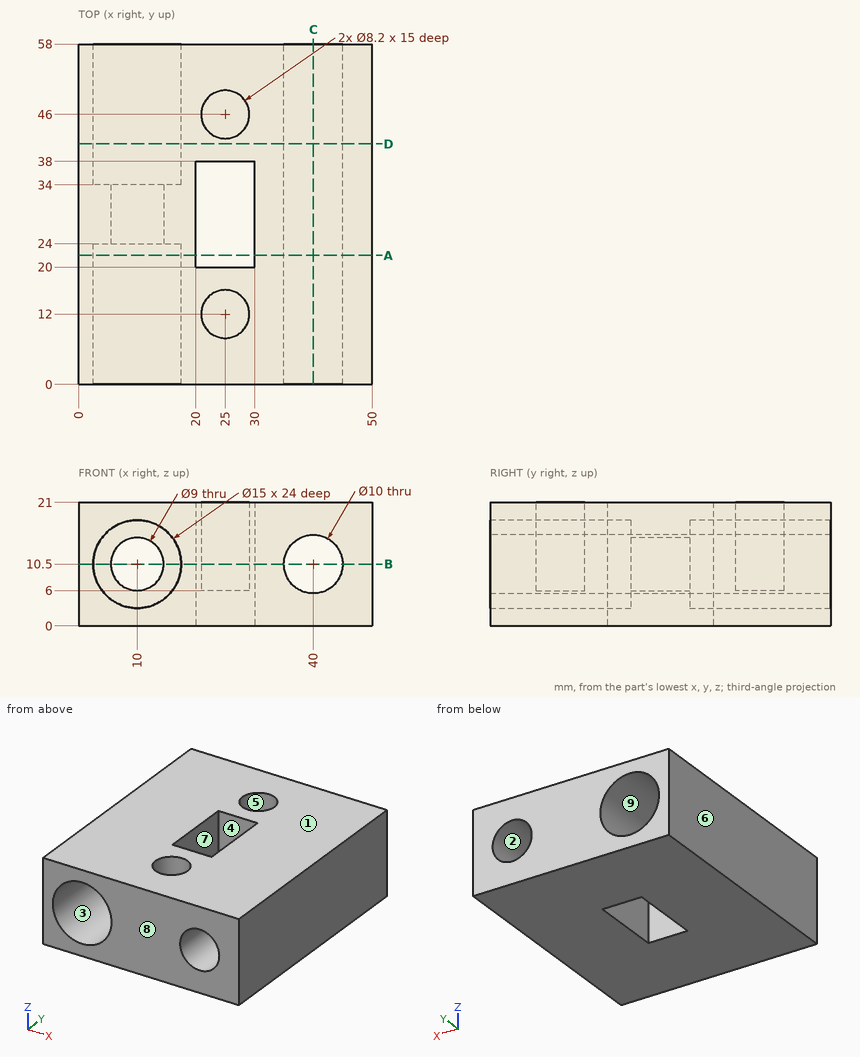
Study the drawing (mm; zero at the part's minimum x, y, z) and answer. A direction names the side the tool comes from. Coordinates: 2 decimals unless noted, no trailing zeros. Write each loop counter-clockwise with the first axis right and the second up, starting at its lowest first coordinate (ties: lowest second). Pieces come first, ordered by that corner, then holes.
Q1. Section D-D, the plane y = 41 is taken. Write down the section's boundary in (x, z), then the cut area to 3 significant figures.
Returned:
outline: (0, 0) - (50, 0) - (50, 21) - (0, 21) - close; hole circle Ø15 at (10, 10.5); hole circle Ø10 at (40, 10.5)
area: 795 mm2
Q2. Section A-A, the plane y = 22 is taken. Write down the section's boundary in (x, z).
Returned:
outline: (0, 0) - (20, 0) - (20, 21) - (0, 21) - close; (30, 0) - (50, 0) - (50, 21) - (30, 21) - close; hole circle Ø15 at (10, 10.5); hole circle Ø10 at (40, 10.5)
Q3. Section C-C, the plane x = 40 is taken. Write down the section's boundary in (y, z).
Returned:
outline: (0, 0) - (58, 0) - (58, 5.5) - (0, 5.5) - close; (0, 15.5) - (58, 15.5) - (58, 21) - (0, 21) - close
Q4. The mould has two halves that part along X. Classify the marked faces 6, 7, 8 and 9: released by +X, released by -X, zero draft, split by the parting line, or undercut.
Returned:
face 6: released by -X
face 7: undercut
face 8: zero draft
face 9: undercut
Q5. Section B-B, the plane z = 10.5 is taken. Write down the section's boundary in (x, y), then the cut area to 3 significant figures.
Returned:
outline: (0, 0) - (2.5, 0) - (2.5, 24) - (5.5, 24) - (5.5, 34) - (2.5, 34) - (2.5, 58) - (0, 58) - close; (14.5, 24) - (17.5, 24) - (17.5, 0) - (35, 0) - (35, 58) - (17.5, 58) - (17.5, 34) - (14.5, 34) - close; (45, 0) - (50, 0) - (50, 58) - (45, 58) - close; hole (20, 20) - (30, 20) - (30, 38) - (20, 38) - close; hole circle Ø8.2 at (25, 12); hole circle Ø8.2 at (25, 46)
area: 1,220 mm2
Q6. Given P1, Ø1.5, axis at x = 9, z = 4.5, coming from the +Y side; P2, Ø2.5, axis at x = 25.5, y = 46, coming from the +Z side; P3, Ø12, axis at x = 10, z = 10.5, coming from the -Y side, each flat-ended and moving along its own axis, determine where each tip first touches the part or whether it passes through.
Returned:
P1: stops at y = 34
P2: stops at z = 6
P3: stops at y = 24
Q7. Which of the six approach directions +Z, -Z, +X, -X, +Y, -Y give full straight-line access (tool end or side, diameter ignored) to the marked faces 1, 2, 3, 4 and 5?
Returned:
face 1: +Z, +X, -X, +Y, -Y
face 2: +Y, -Y
face 3: -Y
face 4: +Z, -Z
face 5: +Z
Q8. Find the intervals of material crossed by line 1 along Y through (x, z) = (25, 12); line 2 along X through (y, z) = (29.75, 10.5); line 3 along Z through (x, y) = (4, 6), in increasing order.
Returned:
line 1: y = 0 to 7.9, 16.1 to 20, 38 to 41.9, 50.1 to 58
line 2: x = 0 to 5.5, 14.5 to 20, 30 to 35, 45 to 50
line 3: z = 0 to 6, 15 to 21
